from build123d import *

# Parameters (mm, degrees)
SKETCH_1_R          = 12
SKETCH_1_R_2        = 2.25
EXTRUDE_1_DEPTH     = 15
SKETCH_2_R          = 13.05
CUT_EXTRUDE_1_DEPTH = 10
SKETCH_3_R          = 2.6
CUT_EXTRUDE_2_DEPTH = 73.5
SKETCH_5_R          = 2.6
CUT_EXTRUDE_3_DEPTH = 10


with BuildPart() as part:
    # 草图1 → 凸台-拉伸1 (new body)
    with BuildSketch(Plane.XY):
        Polygon((-33.800989673, 26.383498279), (-27.44059998, 26.383498279), (-18.800989673, 26.383498279), (-18.800989673, 10.67282016), (22.988332208, -31.116501721), (61.199010327, -31.116501721), (61.199010327, 26.383498279), (76.199010327, 26.383498279), (76.199010327, 41.383498279), (56.199010327, 41.383498279), (-33.800989673, 41.383498279), align=None)
        with Locations((41.199010327, 21.383498279)):
            Circle(SKETCH_1_R, mode=Mode.SUBTRACT)
        with Locations((46.199010327, -21.116501721)):
            Circle(SKETCH_1_R_2, mode=Mode.SUBTRACT)
        with BuildLine():
            Line((-11.126891481, 11.484003342), (3.015244143, 25.626138966))
            ThreePointArc((3.015244143, 25.626138966), (10.086311955, 25.626138966), (10.086311955, 18.555071154))
            Line((10.086311955, 18.555071154), (-4.055823669, 4.41293553))
            Line((-4.055823669, 4.41293553), (-11.126891481, 11.484003342))
        make_face(mode=Mode.SUBTRACT)
    extrude(amount=EXTRUDE_1_DEPTH)

    # 草图2 → 切除-拉伸1 (cut)
    with BuildSketch(Plane(origin=(0, 0, 15), x_dir=(-1, 0, 0), z_dir=(0, 0, -1))):
        with Locations((-41.199010327, 21.383498279)):
            Circle(SKETCH_2_R)
    extrude(amount=CUT_EXTRUDE_1_DEPTH, mode=Mode.SUBTRACT)

    # 草图3 → 切除-拉伸2 (cut, through all)
    with BuildSketch(Plane(origin=(0, 41.383498279, 0), x_dir=(1, 0, 0), z_dir=(0, 1, 0))):
        with Locations((-26.300989673, -7.5)):
            Circle(SKETCH_3_R)
        with Locations((68.699010327, -7.5)):
            Circle(SKETCH_3_R)
    extrude(amount=-CUT_EXTRUDE_2_DEPTH, mode=Mode.SUBTRACT)

    # 草图5 → 切除-拉伸3 (cut)
    with BuildSketch(Plane(origin=(-4.064084756, -4.064084756, 0), x_dir=(0, 0, 1), z_dir=(-0.707106781, -0.707106781, 0))):
        with Locations((7.5, 10.9911308)):
            Circle(SKETCH_5_R)
    extrude(amount=-CUT_EXTRUDE_3_DEPTH, mode=Mode.SUBTRACT)


solid = part.part
Geometry: final body of the model. Coordinates: model frame, mm. A direction names the side the tool comes from. Round coordinates to 2 decimals unless told otherwise and drop trailing zeros. Loops run counter-clockwise (first coordinate to the right, second up) from the corner with the lowest first, then second, coordinate; pieces in that order, holes last. Notation, with made-up numbers: (49, 5) - (88, 5) arc R28 cw to (88, 23) - close; hole circle Ø10 at (38, 34.25). An arc over 180 degrees is marked (long way). Write each question's results on one line, items separated by ' | '. Start each with the question number.
1) First-contact query: P1, Ø15.5, axis at x = 41.2, y = 21.38, coming from the +Z side; P2, Ø6, axis at x = -26.3, z = 7.5, coming from the -Y side; P3, Ø6, axis at x = 9.5, z = 5, coming from the -Y side; P4, Ø5, axis at y = -21.5, z = 13, coming from the +X side. Flat tips, straight axial feed; report the tip coordinate or a pass-through.
2) Cut plane C-C on z = 1.25. Return loops of the section in (x, y), then the cut area to 3 significant figures.
3) Access query for faces 5 (the face through (3.11, 11.58, 7.4)), 6 (the face through (65, 26.383, 7)), 7 (the face through (-30, 26.383, 7)). Directions: +Z, -Z, +X, -X, +Y, -Y. A direction counts if a zero-diameter tool reaches every point of the face in a straight line with its end or side. Return the directions, or none.
4) Cut plane A-A on z = 6.25. Return loops of the section in (x, y).
5) Line query: probe 1 along Y at (x, z) = (41, 4.75); probe 2 along X at (y, z) = (23, 7); probe 3 along X at (y, z) = (24, 3). Output: solid intervals per line, ascending. Write a range as [from, to].
6) Cut plane D-D on x = 9. Return loops of the section in (y, z).
7) Mould query, pull axis Z, two halves, no side actions, for faces 1 (the face through (34.2, 32.4, 10.1)), 2 (the face through (66.1, 34, 7.4)), 3 (the face through (20, 14, 0)), 4 (the face through (-10.3, 6.35, 9.98)). Classes: released by +Z, released by -Z, zero draft, split by the parting line, or undercut.
8) Cut plane B-B on x = 42.5. Return loops of the section in (y, z).
Verdict:
1) P1: passes through | P2: stops at y = 26.38 | P3: stops at y = -20.63 | P4: stops at x = 61.2
2) outline: (-33.8, 26.38) - (-18.8, 26.38) - (-18.8, 10.67) - (22.99, -31.12) - (61.2, -31.12) - (61.2, 26.38) - (76.2, 26.38) - (76.2, 41.38) - (-33.8, 41.38) - close; hole (-11.13, 11.48) - (-4.06, 4.41) - (10.09, 18.56) arc R5 ccw to (3.02, 25.63) - close; hole circle Ø24 at (41.2, 21.38); hole circle Ø4.5 at (46.2, -21.12) | area: 4,670 mm2
3) face 5: +Z, -Z | face 6: +Z, -Z, +X, -Y | face 7: +Z, -Z, -X, -Y
4) outline: (-33.8, 26.38) - (-28.58, 26.38) - (-28.58, 41.38) - (-33.8, 41.38) - close; (-24.02, 26.38) - (-18.8, 26.38) - (-18.8, 10.67) - (-13.45, 5.32) - (-9.21, 9.56) - (-11.13, 11.48) - (3.02, 25.63) arc R5 cw to (10.09, 18.56) - (-4.06, 4.41) - (-5.98, 6.34) - (-10.22, 2.1) - (22.99, -31.12) - (61.2, -31.12) - (61.2, 26.38) - (66.42, 26.38) - (66.42, 41.38) - (-24.02, 41.38) - close; (70.98, 26.38) - (76.2, 26.38) - (76.2, 41.38) - (70.98, 41.38) - close; hole circle Ø26.1 at (41.2, 21.38); hole circle Ø4.5 at (46.2, -21.12)
5) probe 1: y = [-31.12, 9.39], [33.38, 41.38] | probe 2: x = [-18.8, 0.39], [11.47, 28.25], [54.15, 61.2] | probe 3: x = [-18.8, 1.39], [11.17, 29.49], [52.91, 61.2]
6) outline: (-17.13, 0) - (17.47, 0) - (17.47, 15) - (-17.13, 15) - close; (26.45, 0) - (41.38, 0) - (41.38, 15) - (26.45, 15) - close
7) face 1: zero draft | face 2: undercut | face 3: released by -Z | face 4: undercut
8) outline: (-31.12, 0) - (9.45, 0) - (9.45, 5) - (8.4, 5) - (8.4, 15) - (-31.12, 15) - close; (33.31, 0) - (41.38, 0) - (41.38, 15) - (34.37, 15) - (34.37, 5) - (33.31, 5) - close
